```python
from build123d import *

# Parameters (mm, degrees)
SKETCH1_W           = 232.6676516
SKETCH1_H           = 155
BOSS_EXTRUDE1_DEPTH = 1.5875
SKETCH2_R           = 60
CUT_EXTRUDE1_DEPTH  = 204.242095442
SKETCH6_R           = 2.5
CUT_EXTRUDE2_DEPTH  = 204.242095442


with BuildPart() as part:
    # Sketch1 → Boss-Extrude1 (new body)
    with BuildSketch(Plane.XY):
        with Locations((33.576399593, -59.72883635)):
            Rectangle(SKETCH1_W, SKETCH1_H)
    extrude(amount=BOSS_EXTRUDE1_DEPTH)

    # Sketch2 → Cut-Extrude1 (cut, through all)
    with BuildSketch(Plane.XY.offset(1.5875)):
        with Locations((33.576399593, -59.72883635)):
            Circle(SKETCH2_R)
    extrude(amount=-CUT_EXTRUDE1_DEPTH, mode=Mode.SUBTRACT)

    # Sketch6 → Cut-Extrude2 (cut, through all)
    with BuildSketch(Plane.XY.offset(1.5875)):
        with Locations((129.910225393, 10.27116365)):
            Circle(SKETCH6_R)
        with Locations((129.910225393, -129.72883635)):
            Circle(SKETCH6_R)
        with Locations((-62.757426207, 10.27116365)):
            Circle(SKETCH6_R)
        with Locations((-62.757426207, -129.72883635)):
            Circle(SKETCH6_R)
    extrude(amount=-CUT_EXTRUDE2_DEPTH, mode=Mode.SUBTRACT)


solid = part.part
```
Part model, mm, in its own coordinate system. Coordinates: 2 decimals unless noted, no trailing zeros. Loops run counter-clockwise (first coordinate to the right, second up) from the corner with the lowest first, then second, coordinate; pieces in that order, holes last. Notation, with made-up numbers: (-9, 77.25) - (20, 77.25) arc R16 cw to (20, 95.25) - close; hole circle Ø2 at (70, -20). An arc over 180 degrees is marked (long way). Write item = value, one per line. Start each with the question number.
Item 1: Wall check: L1, parallel to Y at x = -65, z = 1.5; L2, parallel to Y at x = -64, z = 1.5; L3, parallel to Y at x = 63, z = 0.6. Give the ranges that are in metal, low to high. Write a range as from..to.
Item 2: Mould opens along X. For faces 1 (the flat face through (-20, -93, 1.588)), 2 (the cylindrical face through (-14.038, -96.238, 0.805)) say: released by +X, released by -X, zero draft, split by the parting line, or undercut.
Item 3: Cut at C-C, the plane z = 0.25. Give the cut face in (x, y).
Item 4: Cut at B-B, the plane x = -13. Give the cut face in (y, z), and give its area (3 significant figures).
Item 5: Cut at A-A, the plane y = -17. Give the cut face in (x, z).
Item 6: Cut at D-D, the plane x = -62.5. Give the cut face in (y, z).
The answers:
q1.L1 = -137.23..-130.83, -128.62..9.17, 11.38..17.77
q1.L2 = -137.23..-131.9, -127.56..8.1, 12.44..17.77
q1.L3 = -137.23..-112.02, -7.44..17.77
q2.face_1 = zero draft
q2.face_2 = undercut
q3.outline = (-82.76, -137.23) - (149.91, -137.23) - (149.91, 17.77) - (-82.76, 17.77) - close; hole circle Ø5 at (-62.76, -129.73); hole circle Ø5 at (-62.76, 10.27); hole circle Ø120 at (33.58, -59.73); hole circle Ø5 at (129.91, -129.73); hole circle Ø5 at (129.91, 10.27)
q4.outline = (-137.23, 0) - (-97.55, 0) - (-97.55, 1.59) - (-137.23, 1.59) - close; (-21.91, 0) - (17.77, 0) - (17.77, 1.59) - (-21.91, 1.59) - close
q4.area = 126 mm2
q5.outline = (-82.76, 0) - (-8.55, 0) - (-8.55, 1.59) - (-82.76, 1.59) - close; (75.7, 0) - (149.91, 0) - (149.91, 1.59) - (75.7, 1.59) - close
q6.outline = (-137.23, 0) - (-132.22, 0) - (-132.22, 1.59) - (-137.23, 1.59) - close; (-127.24, 0) - (7.78, 0) - (7.78, 1.59) - (-127.24, 1.59) - close; (12.76, 0) - (17.77, 0) - (17.77, 1.59) - (12.76, 1.59) - close
